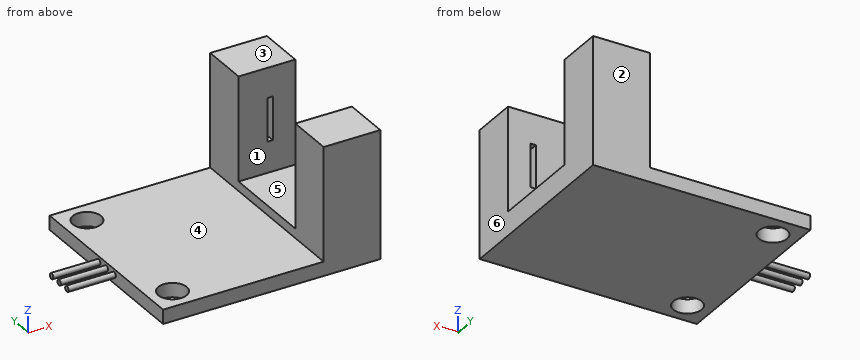
```python
from build123d import *

# Parameters (mm, degrees)
SKETCH_1_W          = 23
SKETCH_1_H          = 20
EXTRUDE_1_DEPTH     = 1.5
SKETCH_2_W          = 6
SKETCH_2_H          = 20
EXTRUDE_2_DEPTH     = 12
SKETCH_3_W          = 6
SKETCH_3_H          = 10
CUT_EXTRUDE_1_DEPTH = 11
SKETCH_4_R          = 0.3
EXTRUDE_3_DEPTH     = 5
SKETCH_5_R          = 1.5
CUT_EXTRUDE_2_DEPTH = 7
SKETCH_6_W          = 0.579660534
SKETCH_6_H          = 4.573153075
CUT_EXTRUDE_3_DEPTH = 2


with BuildPart() as part:
    # 草图1 → 凸台-拉伸1 (new body)
    with BuildSketch(Plane.XY):
        Rectangle(SKETCH_1_W, SKETCH_1_H)
    extrude(amount=EXTRUDE_1_DEPTH)

    # 草图2 → 凸台-拉伸2 (add)
    with BuildSketch(Plane.XY.offset(1.5)):
        with Locations((8.5, 0)):
            Rectangle(SKETCH_2_W, SKETCH_2_H)
    extrude(amount=EXTRUDE_2_DEPTH)

    # 草图3 → 切除-拉伸1 (cut)
    with BuildSketch(Plane.XY.offset(13.5)):
        with Locations((8.5, 0)):
            Rectangle(SKETCH_3_W, SKETCH_3_H)
    extrude(amount=-CUT_EXTRUDE_1_DEPTH, mode=Mode.SUBTRACT)

    # 草图4 → 凸台-拉伸3 (add)
    with BuildSketch(Plane.ZY.offset(11.5)):
        with Locations((0.896688641, 1.343491603)):
            Circle(SKETCH_4_R)
        with Locations((0.896688641, 0)):
            Circle(SKETCH_4_R)
        with Locations((0.896688641, -1.361244933)):
            Circle(SKETCH_4_R)
    extrude(amount=EXTRUDE_3_DEPTH)

    # 草图5 → 切除-拉伸2 (cut)
    with BuildSketch(Plane.XY.offset(1.5)):
        with Locations((-9.028150669, -7.540646778)):
            Circle(SKETCH_5_R)
    cut_extrude_2 = extrude(amount=-CUT_EXTRUDE_2_DEPTH, mode=Mode.SUBTRACT)

    # 镜向1: 切除-拉伸2 across plane
    add(cut_extrude_2.mirror(Plane.ZX), mode=Mode.SUBTRACT)

    # 草图6 → 切除-拉伸3 (cut)
    with BuildSketch(Plane(origin=(0, -5, 0), x_dir=(1, 0, 0), z_dir=(0, 1, 0))):
        with Locations((8.828789431, -8.054724521)):
            Rectangle(SKETCH_6_W, SKETCH_6_H)
    cut_extrude_3 = extrude(amount=-CUT_EXTRUDE_3_DEPTH, mode=Mode.SUBTRACT)

    # 镜向2: 切除-拉伸3 across plane
    add(cut_extrude_3.mirror(Plane.ZX), mode=Mode.SUBTRACT)


solid = part.part
```
CAD build for the part. Positions are in the model's coordinates, mm. Face numbers are marked on the shaded views. A direction names the side the tool comes from. Coordinates: 2 decimals unless noted, no trailing zeros. Write each loop counter-clockwise with the first axis right and the second up, starting at its lowest first coordinate (ties: lowest second). Pieces come first, ordered by that corner, then holes. Notation, with made-up numbers: (0, 39) -> (26, 39) arc R21 cw to (26, 72) -> close; hole circle Ø11 at (-25, -26). An arc over 180 degrees is marked (long way). Use CSV: the item, a comma, the result in double quotes. Start each with the question number.
Item 1: Tool access for the marked faces 4, 5 and 6: list every direction of +Z, -Z, +X, -X, +Y, -Y with a clear straight run to the whole face (end or side of a thin tool).
Item 2: Wall check: probe 1 along Y at (x, z) = (9.25, 11); probe 2 along X at (y, z) = (6.75, 8); probe 3 along X at (y, z) = (3.25, 2.25). Give the ranges that are in metal, low to high.
Item 3: Band-saw the part on C-C, the plane y = 8.25. Write the cut outline in (x, z), plus the area to 3 significant figures.
Item 4: Band-saw the part on A-A, the plane z = 8. Write the cut outline in (x, y).
Item 5: Band-saw the part on D-D, the plane x = -9.75. Write the cut outline in (y, z).
Item 6: Two-plate mould, pull along Y, no slides. Class the marked faces 1, 2 and 3: +Y half, -Y half, draft (parallel to the pull), parting line (faces both ways), or undercut.
Item 7: Band-saw the part on B-B, the plane y = -5.5. Write the cut outline in (x, z).
Item 8: Drop flat-ended pins along their axis: P1, Ø8, axis at y = -3.5, z = 9.5, coming from the -X side; P2, Ø1, axis at x = 6.5, y = -3, coming from the +Z side; P3, Ø5, axis at x = -1.5, y = 4, coming from the +Z side. Give the stop position or say it passes through.
Response values:
1,face 4,"+Z, -X, +Y, -Y"
1,face 5,"+Z, +X, -X"
1,face 6,"+Z, -Z, +X, +Y, -Y"
2,probe 1,"y = -10 to -5, 5 to 10"
2,probe 2,"x = 5.5 to 8.54, 9.12 to 11.5"
2,probe 3,"x = 5.5 to 11.5"
3,outline,"(-11.5, 0) -> (-10.35, 0) -> (-10.35, 1.5) -> (-11.5, 1.5) -> close; (-7.71, 0) -> (11.5, 0) -> (11.5, 13.5) -> (5.5, 13.5) -> (5.5, 1.5) -> (-7.71, 1.5) -> close"
3,area,"103 mm2"
4,outline,"(5.5, -10) -> (11.5, -10) -> (11.5, -5) -> (9.12, -5) -> (9.12, -7) -> (8.54, -7) -> (8.54, -5) -> (5.5, -5) -> close; (5.5, 5) -> (8.54, 5) -> (8.54, 7) -> (9.12, 7) -> (9.12, 5) -> (11.5, 5) -> (11.5, 10) -> (5.5, 10) -> close"
5,outline,"(-10, 0) -> (-8.86, 0) -> (-8.86, 1.5) -> (-10, 1.5) -> close; (-6.23, 0) -> (6.23, 0) -> (6.23, 1.5) -> (-6.23, 1.5) -> close; (8.86, 0) -> (10, 0) -> (10, 1.5) -> (8.86, 1.5) -> close"
6,face 1,"undercut"
6,face 2,"+Y half"
6,face 3,"draft"
7,outline,"(-11.5, 0) -> (11.5, 0) -> (11.5, 13.5) -> (5.5, 13.5) -> (5.5, 1.5) -> (-11.5, 1.5) -> close; hole (8.54, 5.77) -> (9.12, 5.77) -> (9.12, 10.34) -> (8.54, 10.34) -> close"
8,P1,"stops at x = 5.5"
8,P2,"stops at z = 2.5"
8,P3,"stops at z = 1.5"
